from build123d import *

# Parameters (mm, degrees)
BOSS_EXTRUDE1_DEPTH      = 2.58826
M4_CLEARANCE_HOLE1_D     = 4.5
M4_CLEARANCE_HOLE2_D     = 4.5
M4_CLEARANCE_HOLE3_D     = 4.5
M4_CLEARANCE_HOLE3_DEPTH = 12.45
M4_CLEARANCE_HOLE3_TIP   = 1.351936393


with BuildPart() as part:
    # Sketch1 → Boss-Extrude1 (new body)
    with BuildSketch(Plane(origin=(0, 0, 0), x_dir=(1, 0, 0), z_dir=(0, 1, 0))):
        with BuildLine():
            Line((-10, -16), (10, -16))
            Line((10, -16), (10, 1.571108341))
            ThreePointArc((10, 1.571108341), (10.790342052, 8.411859949), (13.119725505, 14.89217598))
            ThreePointArc((13.119725505, 14.89217598), (28.94391879, 35.737554133), (51.350094649, 49.261539007))
            ThreePointArc((51.350094649, 49.261539007), (56.465127412, 50.651730141), (61.744986775, 51.12))
            Line((61.744986775, 51.12), (73, 51.12))
            Line((73, 51.12), (73, 71.65))
            Line((73, 71.65), (60.729747862, 71.65))
            ThreePointArc((60.729747862, 71.65), (57.460315443, 71.516161236), (54.212761864, 71.115540583))
            ThreePointArc((54.212761864, 71.115540583), (18.477348074, 55.823044348), (-6.115833148, 25.722285599))
            ThreePointArc((-6.115833148, 25.722285599), (-9.016876643, 17.34172385), (-10, 8.527908726))
            Line((-10, 8.527908726), (-10, -16))
        make_face()
    extrude(amount=BOSS_EXTRUDE1_DEPTH)

    # M4 Clearance Hole1 (through all)
    with Locations(Plane(origin=(0, 2.58826, 0), x_dir=(1, 0, 0), z_dir=(0, 1, 0))):
        with Locations((-5, 10), (5, 10), (5, -10), (-5, -10)):
            Hole(M4_CLEARANCE_HOLE1_D / 2)

    # M4 Clearance Hole2 (through all)
    with Locations(Plane(origin=(0, 2.58826, 0), x_dir=(1, 0, 0), z_dir=(0, 1, 0))):
        with Locations((61, 66.385), (68, 56.385)):
            Hole(M4_CLEARANCE_HOLE2_D / 2)

    # M4 Clearance Hole3
    with Locations(Plane(origin=(0, 0, 0), x_dir=(-1, 0, 0), z_dir=(0, -1, 0))):
        with Locations((-45, 51.65)):
            Hole(M4_CLEARANCE_HOLE3_D / 2, depth=M4_CLEARANCE_HOLE3_DEPTH)
            with Locations((0, 0, -(M4_CLEARANCE_HOLE3_DEPTH + M4_CLEARANCE_HOLE3_TIP / 2))):  # 118° drill point
                Cone(0, M4_CLEARANCE_HOLE3_D / 2, M4_CLEARANCE_HOLE3_TIP, mode=Mode.SUBTRACT)


solid = part.part
Source: CAD feature listing. Evaluate the final solid. Frame: model axes, mm. A direction names the side the tool comes from. Give positions to 0.01 mm unless a question says otherwise; leave off trailing zeros. Write each loop counter-clockwise with the first axis right and the second up, starting at its lowest first coordinate (ties: lowest second). Pieces come first, ordered by that corner, then holes. Notation, with made-up numbers: M 39,82 L 90,82 A20 cw 90,100 Z; hole C 85,60 d6. An arc over 180 degrees is marked long. Return JSON: item names as keys, results as strings. Group by question number.
1) Cut plane C-C, the plane y = 0.4. Output: boundary loops of the cut face in (x, z) (3 decimals), plus the area to 3 significant figures.
2) Cut plane B-B, the plane x = 45. Output: boundary loops of the cut face in (y, z), plus the area to 3 significant figures.
3) Set-up query: faces 1 (the face through (10, 1, 7)), 2 (the face through (-6.21, 1.276, 8.103)). Return all of +Z, -Z, +X, -X, +Y, -Y with unobstructed straight access to the full face (end or side cutting, diameter ignored); none if empty.
4) Cut plane D-D, the plane x = -5. Output: boundary loops of the cut face in (y, z).
5) Pull-direction query (Z, two-part tool) for faces 3 (the face through (-8.99, 1.28, -17.46)), 4 (the face through (63.248, 1.276, -66.484)), 5 (the face through (22, 2.588, -35)); classes: pulls with the +Z half, pulls with the -Z half, needs draft (parallel to the pull), parting line crosses it, or undercut.
6) Pin query (flat end, axial travel): P1, Ø1, axis at x = 10.5, y = 2, coming from the -Z side; P2, Ø0.8, axis at x = 67, y = 1.5, coming from the +Z side; P3, Ø1.3, axis at y = 1.5, z = 10.5, coming from the +X side. Return the tip coordinate at first contact, or that it passes through.
7) Cut plane A-A, the plane z = 10. Output: boundary loops of the cut face in (x, y), plus the area to 3 significant figures.
8) Material intervals for line 1 along X through (y, z) = (0.9, 10); line 2 along X through (y, z) = (0.9, -10); line 3 along Z through (x, y) = (61, 0.75) (3 decimals), sorted ascending. Write a range as [from, to].
Recorded:
{
 "1": {"outline": "M -10,-8.528 A40 ccw -6.116,-25.722 A81.528 ccw 54.213,-71.116 A40 ccw 60.73,-71.65 L 73,-71.65 L 73,-51.12 L 61.745,-51.12 A30 cw 51.35,-49.262 A69.571 cw 13.12,-14.892 A30 cw 10,-1.571 L 10,16 L -10,16 Z; hole C -5,-10 d4.5; hole C -5,10 d4.5; hole C 5,-10 d4.5; hole C 5,10 d4.5; hole C 45,-51.65 d4.5; hole C 61,-66.385 d4.5; hole C 68,-56.385 d4.5", "area": "2,500 mm²"},
 "2": {"outline": "M 0,-69.04 L 2.59,-69.04 L 2.59,-53.9 L 0,-53.9 Z; M 0,-49.4 L 2.59,-49.4 L 2.59,-46.55 L 0,-46.55 Z", "area": "46.6 mm²"},
 "3": {"face 1": "+Z, +X, +Y, -Y", "face 2": "+Y, -Y"},
 "4": {"outline": "M 0,-27.98 L 2.59,-27.98 L 2.59,-12.25 L 0,-12.25 Z; M 0,-7.75 L 2.59,-7.75 L 2.59,7.75 L 0,7.75 Z; M 0,12.25 L 2.59,12.25 L 2.59,16 L 0,16 Z"},
 "5": {"face 3": "pulls with the -Z half", "face 4": "undercut", "face 5": "needs draft"},
 "6": {"P1": "stops at z = -49.46", "P2": "stops at z = -51.12", "P3": "stops at x = 10"},
 "7": {"outline": "M -10,0 L -7.25,0 L -7.25,2.59 L -10,2.59 Z; M -2.75,0 L 2.75,0 L 2.75,2.59 L -2.75,2.59 Z; M 7.25,0 L 10,0 L 10,2.59 L 7.25,2.59 Z", "area": "28.5 mm²"},
 "8": {"line 1": "x = [-10, -7.25], [-2.75, 2.75], [7.25, 10]", "line 2": "x = [-9.97, -7.25], [-2.75, 2.75], [7.25, 11.21]", "line 3": "z = [-71.65, -68.635], [-64.135, -51.111]"}
}
